Source: CAD feature listing. Evaluate the final solid. Frame: model axes, mm. Face numbers are marked on the shaded views. A direction names the side the tool comes from. Give positions to 0.01 mm unless a question says otherwise; leave off trailing zeros. Order: outer loops, then holes, each group sorted by start corner. A loop starts at its lowest first (then second) coordinate and runs counter-clockwise, first axis right, second up.
1) Section C-C, the plane y = 20. Return loops of the section in (x, z).
2) First-contact query: P1, Ø1, axis at x = -1.5, y = 17.5, coming from the -Z side; P2, Ø1.9, axis at x = 4, z = 5.5, coming from the -Y side; P3, Ø3, axis at x = 7.5, y = 18, coming from the -Z side; P4, Ø1.5, axis at x = 6.5, z = -2, coming from the +Y side. Flat tips, straight axial feed; report the tip coordinate or a pass-through.
3) Material intervals for line 1 (Z direction, x = 3.75, y = 2.05); line 2 (Y direction, x = 2.25, z = -9); line 3 (X direction, y = 4, z = 5.25), sorted ascending.
4) Section D-D, the plane x = 10. Return loops of the section in (y, z).
5) Access query for the marked faces 4, 5 and 6. Directions: +Z, -Z, +X, -X, +Y, -Y. A direction counts if a zero-diameter tool reaches every point of the face in a straight line with its end or side. Return the directions, or none.
6) Section A-A, the plane y = 29. Return loops of the section in (x, z).
7) Section B-B, the plane z = 5. Return loops of the section in (x, y).
8) Draft query along Z for the marked faces 1, 2 and 3. Return one class per face: released by +Z, released by -Z, zero draft, split by the parting line, or undercut.
```python
from build123d import *

# Parameters (mm, degrees)
BOSS_EXTRUDE2_DEPTH            = 5
SKETCH3_R                      = 4
BOSS_EXTRUDE3_DEPTH            = 22.5
SKETCH4_R                      = 3
BOSS_EXTRUDE4_DEPTH            = 2
SKETCH5_R                      = 4
BOSS_EXTRUDE5_DEPTH            = 2
SKETCH7_W                      = 1.89865
SKETCH7_H                      = 5
F_6_CLEARANCE_HOLE1_AT_2_COUNT = 2
F_6_CLEARANCE_HOLE1_AT_2_PITCH = 11.930689284


with BuildPart() as part:
    # Sketch2 → Boss-Extrude2 (new body)
    with BuildSketch(Plane(origin=(0, 0, 0), x_dir=(1, 0, 0), z_dir=(0, 1, 0))):
        with BuildLine():
            ThreePointArc((-1.921673483, -7.798539123), (3.967844549, -11.837003018), (9.548776015, -7.381801872))
            Line((9.548776015, -7.381801872), (10.998470019, -1.926053578))
            ThreePointArc((10.998470019, -1.926053578), (11.24988985, -0.04064778), (11.018921171, 1.84737246))
            Line((11.018921171, 1.84737246), (9.565136937, 7.567628243))
            ThreePointArc((9.565136937, 7.567628243), (3.75, 12.089730275), (-2.065136937, 7.567628243))
            Line((-2.065136937, 7.567628243), (-3.518921171, 1.84737246))
            ThreePointArc((-3.518921171, 1.84737246), (-3.749830525, -0.050419155), (-3.493426606, -1.944934706))
            Line((-3.493426606, -1.944934706), (-1.921673483, -7.798539123))
        make_face()
    extrude(amount=BOSS_EXTRUDE2_DEPTH)

    # Sketch3 → Boss-Extrude3 (add)
    with BuildSketch(Plane(origin=(0, 5, 0), x_dir=(1, 0, 0), z_dir=(0, 1, 0))):
        with Locations(Location((3.75, -5.840959009, 0), (0, 0, 90))):
            Circle(SKETCH3_R)
        with Locations(Location((3.75, 6.089730275, 0), (0, 0, 90))):
            Circle(SKETCH3_R)
    extrude(amount=BOSS_EXTRUDE3_DEPTH)

    # Sketch4 → Boss-Extrude4 (add)
    with BuildSketch(Plane(origin=(0, 27.5, 0), x_dir=(1, 0, 0), z_dir=(0, 1, 0))):
        with Locations(Location((3.75, -5.840959009, 0), (0, 0, 270))):
            Circle(SKETCH4_R)
        with Locations(Location((3.75, 6.089730275, 0), (0, 0, 270))):
            Circle(SKETCH4_R)
    extrude(amount=BOSS_EXTRUDE4_DEPTH)

    # Sketch5 → Boss-Extrude5 (add)
    with BuildSketch(Plane(origin=(0, 29.5, 0), x_dir=(1, 0, 0), z_dir=(0, 1, 0))):
        with Locations(Location((3.75, -5.840959009, 0), (0, 0, 90))):
            Circle(SKETCH5_R)
        with Locations(Location((3.75, 6.089730275, 0), (0, 0, 90))):
            Circle(SKETCH5_R)
    extrude(amount=BOSS_EXTRUDE5_DEPTH)

    # Sketch7 → #6 Clearance Hole1 (revolve, cut)
    with BuildSketch(Plane(origin=(3.75, 5, -6.089730275), x_dir=(0, 0, 1), z_dir=(1, 0, 0))):
        with Locations((0.949325, 2.5)):
            Rectangle(SKETCH7_W, SKETCH7_H)
    f_6_clearance_hole1 = revolve(axis=Axis((3.75, 11.35, -6.089730275), (0, -1, 0)), mode=Mode.SUBTRACT)

    # #6 Clearance Hole1 at 2: #6 Clearance Hole1 ×2
    with Locations(*[(0, 0, i * F_6_CLEARANCE_HOLE1_AT_2_PITCH) for i in range(1, F_6_CLEARANCE_HOLE1_AT_2_COUNT)]):
        add(f_6_clearance_hole1, mode=Mode.SUBTRACT)


solid = part.part
```
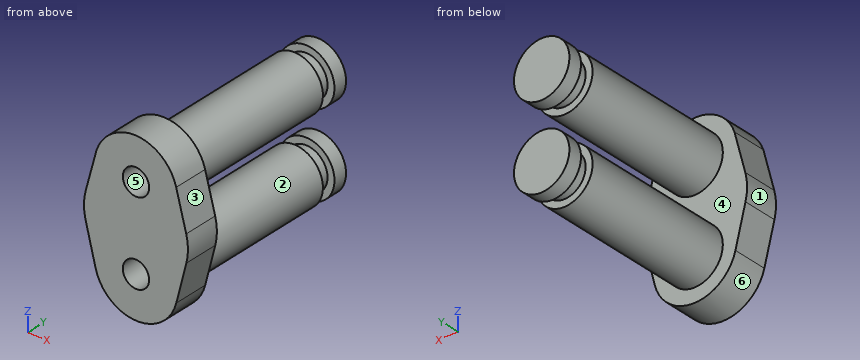
From the geometry:
1. outline: circle Ø8 at (3.75, -6.09); circle Ø8 at (3.75, 5.84)
2. P1: passes through
2. P2: stops at y = 5
2. P3: stops at z = -9.4
2. P4: stops at y = 5
3. line 1: z = -12.09 to -7.99, -4.19 to 3.94, 7.74 to 11.84
3. line 2: y = 0 to 27.5, 29.5 to 31.5
3. line 3: x = -2.61 to 1.95, 5.55 to 10.12
4. outline: (0, -5.86) - (5, -5.86) - (5, 5.68) - (0, 5.68) - close
5. face 4: +Y
5. face 5: -Y
5. face 6: -Z, +Y, -Y
6. outline: circle Ø6 at (3.75, -6.09); circle Ø6 at (3.75, 5.84)
7. outline: (-2.67, 0) - (2.05, 0) - (2.05, 5) - (5.45, 5) - (5.45, 0) - (10.18, 0) - (10.18, 5) - (7.66, 5) - (7.66, 27.5) - (6.63, 27.5) - (6.63, 29.5) - (7.66, 29.5) - (7.66, 31.5) - (-0.16, 31.5) - (-0.16, 29.5) - (0.87, 29.5) - (0.87, 27.5) - (-0.16, 27.5) - (-0.16, 5) - (-2.67, 5) - close
8. face 1: split by the parting line
8. face 2: undercut
8. face 3: released by +Z
